Read the model definition and answer for the solid it produces. Units are mm, in the model's axes. A direction names the side the tool comes from. Coordinates: 2 decimals unless noted, no trailing zeros. Loops run counter-clockwise (first coordinate to the right, second up) from the corner with the lowest first, then second, coordinate; pieces in that order, holes last. Notation, with made-up numbers: M 49.25,54 L 99.25,54 A21 cw 99.25,80 Z; hole C 48.25,-20.75 d4. An arc over 180 degrees is marked long. Put each result on its own line as item: value.
Autodesk Inventor part; units mm, degrees
ref_plane "YZ Plane" through (0, 0, 0) normal (1, 0, 0) x (0, 1, 0)
ref_plane "XZ Plane" through (0, 0, 0) normal (0, 1, 0) x (-1, 0, 0)
ref_plane "XY Plane" through (0, 0, 0) normal (0, 0, 1) x (1, 0, 0)
sketch "Szkic2" plane through (0, 0, 0) normal (1, 0, 0) x (0, 1, 0)
  line L0 (0, -2.9) -> (0, 2.9)
  line L1 (-1.5, -1.5) -> (-1.5, 1.5)
  line L2 (-1.5, -1.5) -> (0, -2.9)
  line L3 (-1.5, 1.5) -> (0, 2.9)
  line L4 (0, 0) -> (-12, 0)
  line L5 (-12, 0) -> (-12, -1.5)
  line L6 (-12, -1.5) -> (-1.5, -1.5)
  dimension "d0" = 5.8
  dimension "d2" = 3
  dimension "d3" = 1.5
  dimension "d4" = 12
  dimension "d5" = 1.5
revolve "Obrót1" add sketch "Szkic2" angle 360 about axis through (0, 0, 0) along (0, -1, 0) contours L2 L1 L4 L0 | L6 L5 L4 L1
sketch "Szkic3" plane through (0, 0, 0) normal (0, 1, 0) x (1, 0, 0)
  line L0 (-1.1673, -0.633) -> (-1.1318, 0.6945)
  line L1 (-1.1318, 0.6945) -> (0.0355, 1.3274)
  line L2 (0.0355, 1.3274) -> (1.1673, 0.633)
  line L3 (1.1673, 0.633) -> (1.1318, -0.6945)
  line L4 (1.1318, -0.6945) -> (-0.0355, -1.3274)
  line L5 (-0.0355, -1.3274) -> (-1.1673, -0.633)
  point P0 (0, 0)
  point P1 (0, 0)
  dimension "d7" = 2.3
extrude "Wyciągnięcie proste1" cut sketch "Szkic3" against normal blind 2
fillet "Zaokrąglenie1" radius 0.5 6 edges at (-1.1496, -2, -0.0308) (-0.6014, -2, 0.9802) (-0.5482, -2, -1.011) (0.6014, -2, -0.9802) (0.5482, -2, 1.011) (1.1496, -2, 0.0308)
fillet "Zaokrąglenie2" radius 0.5 1 edges at (0, -1.5, 1.5)
fillet "Zaokrąglenie3" radius 0.1 1 edges at (0, 0, 2.9)
thread "Gwint1"
chamfer "Faza1" distance 0.5 angle 45 1 edges at (0, -12, 1.5)
properties part number "Screw M3 12mm flat head"
1) Which of the six approach directions +Z, -Z, +X, -X, +Y, -Y give full straight-line access (tool end or side, diameter ignored) to faces 4 (the flat face through (0.556, -0.74, 1.007)), 5 (the flat face through (-1, 0, -1))?
Answer list:
face 4: +Y
face 5: +Z, -Z, +X, -X, +Y
2) Given pin 1 Ø1 at (x, z) = (-1, -1.5) entering from -Y; pin 2 Ø3 at (x, y) = (1, -10) entering from -Z; pin 3 Ø3 at (y, z) = (-10, 2) entering from +X, each flat-ended and moving along its own axis, determine where each tip first touches the part or whether it passes through.
Answer list:
pin 1: stops at y = -11.7
pin 2: stops at z = -1.5
pin 3: stops at x = 1.41
3) Find section A-A, the plane y = -5. Write down the section's boundary in (x, z), plus the area to 3 significant figures.
Answer list:
outline: C 0,0 d3
area: 7.07 mm^2
4) Determine the mould class of faces 1 (the flat face through (0, -2, 0)), 2 (the cylindrical face through (-0.07, -6.53, 1.5)), 3 (the flat face through (0, -12, 0)) for opening direction X: released by +X, released by -X, zero draft, split by the parting line, or undercut.
Answer list:
face 1: undercut
face 2: split by the parting line
face 3: zero draft
5) Straight lines are drawn through the part: line 1 (Z direction, x = -0.1, y = -9.25); line 2 (Z direction, x = -1.3, y = -3); line 3 (X direction, y = -1, z = 0.1). For each, find the intervals that lie inside material, in ascending order. Write a range as [from, to].
Answer list:
line 1: z = [-1.5, 1.5]
line 2: z = [-0.75, 0.75]
line 3: x = [-1.96, -1.15], [1.15, 1.96]
